Autodesk Inventor part; units mm, degrees
ref_plane "YZ Plane" through (0, 0, 0) normal (1, 0, 0) x (0, 1, 0)
ref_plane "XZ Plane" through (0, 0, 0) normal (0, 1, 0) x (-1, 0, 0)
ref_plane "XY Plane" through (0, 0, 0) normal (0, 0, 1) x (1, 0, 0)
sketch "Sketch1" plane through (0, 0, 0) normal (0, 0, 1) x (1, 0, 0)
  line L0 (-190.5, -317.5) -> (190.5, -317.5)
  line L1 (190.5, -317.5) -> (190.5, 0)
  line L2 (-190.5, -317.5) -> (-190.5, 0)
  arc A0 (190.5, 0) -> (-190.5, 0) centre (0, 0) ccw
  dimension "d0" = 508
  dimension "d1" = 381
extrude "Extrusion1" add sketch "Sketch1" along normal blind 9.525
hole "Hole1" at (82.55, -241.3, 9.525) direction (0, 0, -1) diameter 7.9375 depth 25.4 tip angle 118
hole "Hole2" at (-82.55, -241.3, 9.525) direction (0, 0, -1) diameter 7.9375 depth 25.4 tip angle 118
hole "Hole3" at (82.55, -104.775, 9.525) direction (0, 0, -1) diameter 7.9375 depth 25.4 tip angle 118
hole "Hole4" at (-82.55, -104.775, 9.525) direction (0, 0, -1) diameter 7.9375 depth 25.4 tip angle 118
hole "Hole5" at (-82.55, 101.6, 9.525) direction (0, 0, -1) diameter 7.9375 depth 25.4 tip angle 118
hole "Hole6" at (82.55, 101.6, 9.525) direction (0, 0, -1) diameter 7.9375 depth 25.4 tip angle 118
hole "Hole7" at (0, 25.4, 9.525) direction (0, 0, -1) diameter 212.725 depth 25.4 tip angle 118
properties part number "Top_Deck"
Source: CAD feature listing. Evaluate the final solid. Frame: model axes, mm. Give positions to 0.01 mm unless a question says otherwise; leave off trailing zeros. Loops run counter-clockwise (first coordinate to the right, second up) from the corner with the lowest first, then second, coordinate; pieces in that order, holes last. Notation, with made-up numbers: (65, 22.5) -> (122, 22.5) arc R11 ccw to (122, 27.5) -> close; hole circle Ø6 at (-20, -33.75). An arc over 180 degrees is marked (long way). Use a Markdown table: item, result. Add a question column.
(1) Pull-direction query (Y, two-part tool) for faces 1 (the face through (-31.95, -76.05, 4.7)), 2 (the face through (-3, -116, 0)), 3 (the face through (-4.189, 190.454, 4.696)); classes: +Y half, -Y half, draft (parallel to the pull), parting line (faces both ways), or undercut.
(2) Section query A-A (z = 1.75). Count the separate pieces of the cut face and the enclosed holes in it, then the cut area to 3 significant figures.
(3) Ray query, line 1 (X direction, y = -241.3, z = 2); line 2 (Y direction, x = 0, z = 6); line 3 (Y direction, x = 82.55, z = 3). Return the intervals inside material, ascending.
(4) Section query B-B (x = 0). Output: boundary loops of the cut face in (y, z) (1 decimal).
(5) Section query C-C (y = 25.4). Output: boundary loops of the cut face in (x, z) (1 decimal).
(6) Section query D-D (x = -139). Output: boundary loops of the cut face in (y, z) (3 decimals), then the cut area to 3 significant figures.
(7) First-contact query: pin 1 Ø5 at (x, y) = (82.55, -104.775) entering from -Z; pin 2 Ø10.5 at (x, y) = (-82.55, 101.6) entering from +Z (3 decimals); pin 3 Ø2 at (x, z) = (-25.5, 2.5) entering from +Y; pin 4 Ø2 at (x, z) = (73, 2.5) entering from +Y. Flat tips, straight axial feed; report the tip coordinate or a pass-through.
Checked values:
| question | item | result |
|---|---|---|
| 1 | face 1 | undercut |
| 1 | face 2 | draft |
| 1 | face 3 | +Y half |
| 2 | separate pieces | 1 |
| 2 | enclosed holes | 7 |
| 2 | area | 142,000 mm^2 |
| 3 | line 1 | -190.5 to -86.52, -78.58 to 78.58, 86.52 to 190.5 |
| 3 | line 2 | -317.5 to -80.96, 131.76 to 190.5 |
| 3 | line 3 | -317.5 to -245.27, -237.33 to -108.74, -100.81 to -41.67, 92.47 to 97.63, 105.57 to 171.69 |
| 4 | outline | (-317.5, 0) -> (-81, 0) -> (-81, 9.5) -> (-317.5, 9.5) -> close; (131.8, 0) -> (190.5, 0) -> (190.5, 9.5) -> (131.8, 9.5) -> close |
| 5 | outline | (-188.8, 0) -> (-106.4, 0) -> (-106.4, 9.5) -> (-188.8, 9.5) -> close; (106.4, 0) -> (188.8, 0) -> (188.8, 9.5) -> (106.4, 9.5) -> close |
| 6 | outline | (-317.5, 0) -> (130.266, 0) -> (130.266, 9.525) -> (-317.5, 9.525) -> close |
| 6 | area | 4,260 mm^2 |
| 7 | pin 1 | through |
| 7 | pin 2 | z = 9.525 |
| 7 | pin 3 | y = 188.92 |
| 7 | pin 4 | y = 176.37 |
